The model under review builds one solid part; all positions refer to its coordinate system, in mm. A direction names the side the tool comes from. Coordinates: 2 decimals unless noted, no trailing zeros.
Autodesk Inventor part; units mm, degrees
ref_plane "Work Plane1" through (-14, 16, -288) normal (0, 1, 0) x (1, 0, 0)
ref_plane "YZ Plane" through (0, 0, 0) normal (1, 0, 0) x (0, 1, 0)
ref_plane "XY Plane" through (0, 0, 0) normal (0, 0, 1) x (1, 0, 0)
sketch "Sketch1" plane through (0, 0, 0) normal (0, 1, 0) x (-1, 0, 0)
  point P0 (0, 0)
ref_plane "Work Plane1" through (-14, 16, -288) normal (0, 1, 0) x (1, 0, 0)
sketch "Sketch3" plane through (0, 0, 0) normal (0, 1, 0) x (-1, 0, 0)
  line L0 (14, 0) -> (-14, 0)
  line L1 (14, -144) -> (14, 0)
  line L2 (-14, -144) -> (-14, 0)
  circle A0 centre (5.66, -138.34) radius 1.85
  circle A1 centre (-5.66, -138.34) radius 1.85
  circle A2 centre (0, -136) radius 1.85
  circle A3 centre (-5.66, -74.34) radius 1.85
  circle A4 centre (-5.66, -85.66) radius 1.85
  circle A5 centre (5.66, -85.66) radius 1.85
  circle A6 centre (5.66, -74.34) radius 1.85
  circle A7 centre (8, -80) radius 1.85
  circle A8 centre (-8, -80) radius 1.85
  circle A9 centre (0, -72) radius 1.85
  circle A10 centre (0, -88) radius 1.85
  circle A11 centre (0, -80) radius 4
  circle A12 centre (8, -112) radius 1.85
  circle A13 centre (-8, -112) radius 1.85
  circle A14 centre (0, -104) radius 1.85
  circle A15 centre (0, -120) radius 1.85
  circle A16 centre (0, -112) radius 4
  circle A17 centre (-5.66, -10.34) radius 1.85
  circle A18 centre (-5.66, -21.66) radius 1.85
  circle A19 centre (5.66, -21.66) radius 1.85
  circle A20 centre (5.66, -10.34) radius 1.85
  circle A21 centre (8, -16) radius 1.85
  circle A22 centre (-8, -16) radius 1.85
  circle A23 centre (0, -8) radius 1.85
  circle A24 centre (0, -24) radius 1.85
  circle A25 centre (0, -16) radius 4
  circle A26 centre (8, -48) radius 1.85
  circle A27 centre (-8, -48) radius 1.85
  circle A28 centre (0, -40) radius 1.85
  circle A29 centre (0, -56) radius 1.85
  circle A30 centre (0, -48) radius 4
  circle A31 centre (0, -128) radius 4
  circle A32 centre (0.1754, -96) radius 4
  circle A33 centre (0, -64) radius 4
  circle A34 centre (0, -32) radius 4
  line L3 (14, -144) -> (-14, -144)
  point P0 (0, 0)
extrude "Extrusion1" add sketch "Sketch3" along normal blind 3.175
sketch "Sketch4" plane through (0, 0, 0) normal (0, -1, 0) x (1, 0, 0)
  point P0 (0, 0)
sketch "Sketch10" plane through (-14, 0, 0) normal (0, 0, 1) x (1, 0, 0)
  line L0 (0, 0) -> (28, 0)
  line L1 (0, 0) -> (82.55, 0)
  line L2 (82.55, 0) -> (82.55, 69.85)
  line L3 (0, 3.175) -> (28, 3.175)
  line L4 (28, 0) -> (28, 3.175)
  line L5 (0, 0) -> (0, 3.175)
  line L6 (0, 0) -> (-12.7, 0)
  line L7 (-12.7, 3.175) -> (0, 3.175)
  line L8 (0, 3.175) -> (0, 0)
  arc A0 (-3.0407, 3.175) -> (82.55, 64.0105) centre (-82.4635, 205.5441) ccw
  arc A1 (-12.7, 3.175) -> (82.55, 69.85) centre (-103.2617, 233.9221) ccw
  line L9 (-12.7, 3.175) -> (-12.7, 0)
  point P0 (14, 0)
  dimension "d18" = 82.55
  dimension "d19" = 69.85
extrude "Extrusion7" add sketch "Sketch10" against normal up to surface (144 mm away) contours L6 L9 L7 L5 | L7 A1 L2 A0
fillet "Fillet3" radius 1.016 1 edges at (-17.0407, 3.175, -72)
sketch "Sketch11" plane through (0, 0, 0) normal (0, -1, 0) x (1, 0, 0)
  line L0 (-26.7, 0) -> (14, 0)
  line L1 (-26.7, 0) -> (-26.7, -144)
  line L2 (14, -144) -> (-26.7, -144)
  line L3 (14, 0) -> (14, -144)
  circle A0 centre (0, -32) radius 4
  circle A1 centre (-0.1754, -96) radius 4
  circle A2 centre (0, -48) radius 4
  circle A3 centre (0, -40) radius 1.85
  circle A4 centre (-8, -48) radius 1.85
  circle A5 centre (0, -8) radius 1.85
  circle A6 centre (-8, -16) radius 1.85
  circle A7 centre (0, -120) radius 1.85
  circle A8 centre (8, -112) radius 1.85
  circle A9 centre (-5.66, -138.34) radius 1.85
  circle A10 centre (5.66, -138.34) radius 1.85
  circle A11 centre (0, -136) radius 1.85
  circle A12 centre (-8, -80) radius 1.85
  circle A13 centre (8, -80) radius 1.85
  circle A14 centre (0, -72) radius 1.85
  circle A15 centre (0, -88) radius 1.85
  circle A16 centre (-8, -112) radius 1.85
  circle A17 centre (0, -104) radius 1.85
  circle A18 centre (0, -112) radius 4
  circle A19 centre (8, -16) radius 1.85
  circle A20 centre (0, -24) radius 1.85
  circle A21 centre (8, -48) radius 1.85
  circle A22 centre (0, -56) radius 1.85
  circle A23 centre (0, -128) radius 4
  circle A24 centre (0, -64) radius 4
  circle A25 centre (0, -16) radius 4
  circle A26 centre (-5.66, -10.34) radius 1.85
  circle A27 centre (-5.66, -21.66) radius 1.85
  circle A28 centre (5.66, -21.66) radius 1.85
  circle A29 centre (5.66, -10.34) radius 1.85
  circle A30 centre (0, -80) radius 4
  circle A31 centre (-5.66, -74.34) radius 1.85
  circle A32 centre (-5.66, -85.66) radius 1.85
  circle A33 centre (5.66, -85.66) radius 1.85
  circle A34 centre (5.66, -74.34) radius 1.85
  point P0 (0, 0)
extrude "Extrusion8" add sketch "Sketch11" along normal blind 6.35
ref_plane "Work Plane2" through (68.55, 64.0105, 12.7) normal (0, 0, 1) x (1, 0, 0)
mirror "Mirror1" about plane through (68.55, 64.0105, 12.7) normal (0, 0, 1) of "Extrusion1", "Extrusion7", "Fillet3", "Extrusion8"
sketch "Sketch13" plane through (0, -6.35, 0) normal (0, -1, 0) x (1, 0, 0)
  line L0 (-71.1109, -172.9403) -> (93.8528, -172.9403)
  line L1 (93.8528, -172.9403) -> (93.8528, 6.9583)
  line L2 (93.8528, 6.9583) -> (-71.1109, 6.9583)
  line L3 (-71.1109, 6.9583) -> (-71.1109, -172.9403)
  point P0 (0, 0)
extrude "Extrusion10" cut sketch "Sketch13" against normal blind 381
properties part number "rampside1"
(1) Machinability: for faces 5 (the face through (68.55, 67, 96)), 6 (the face through (32.16, 30.28, 96.39)), 7 (the face through (14, -2, 98)), which of the approach directions +Z, -Z, +X, -X, +Y, -Y give a long, thin tool a straight path to every point of the face, cutting with its end or side? Answer none if there is none.
A:
face 5: +Z, -Z, +X, +Y, -Y
face 6: +Z, -Z, +X
face 7: +Z, -Z, +X, -Y
(2) Wall thickness on probe 1 along X at (y, z) = (1.4, 99.74); probe 2 along X at (y, z) = (2.05, 73.4); probe 3 along Z at (x, y) = (-5.66, 2.25): over which ranges is each line inside the solid? List them lowest first.
A:
probe 1: x = -26.7 to -7.51, -3.81 to 3.81, 7.51 to 14
probe 2: x = -26.7 to -9.85, -6.15 to -4, 4 to 6.15, 9.85 to 14
probe 3: z = 25.4 to 33.89, 37.59 to 45.21, 48.91 to 97.89, 101.59 to 109.21, 112.91 to 161.89, 165.59 to 169.4
(3) For pin 1 Ø4.5 at (x, z) = (0, 33.4) entering from +Y; pin 2 Ø4 at (x, z) = (-15.5, 149.5) entering from +Y; pin 3 Ø4 at (y, z) = (32.5, 43) entering from +X, all flat-tipped, find the tip position at first contact; note any pin that passes through.
A:
pin 1: stops at y = 16.75
pin 2: stops at y = 8.8
pin 3: stops at x = 37.72
(4) Draft analysis for pull direction Y (two halves, no side actions). For faces 1 (the face through (4, 3.175, 96)), 2 (the face through (-6, -6.35, 96)), 3 (the face through (10, 18, 169.4)), 4 (the face through (25.56, 31.32, 96.39)), state which applies: released by +Y, released by -Y, zero draft, split by the parting line, or undercut.
A:
face 1: undercut
face 2: released by -Y
face 3: zero draft
face 4: released by +Y
(5) We need section B-B, the plane z = 105.4. Count the separate pieces of the cut face and the enclosed holes in it, and give its area (3 significant figures).
A:
separate pieces: 4
enclosed holes: 0
area: 731 mm2
